Job drawing, mm, ordinate dimensions from the low corner. One solid piece. A direction names the side the tool comes from. Round coordinates to 2 decimals unless told otherwise and drop trailing zeros. Write each loop counter-clockwise with the first axis right and the second up, starting at its lowest first coordinate (ties: lowest second). Pieces come first, ordered by that corner, then holes. Notation, with made-up numbers: M 72.5,16.5 L 86.5,16.5 A34 ccw 86.5,54.5 Z; hole C 13,88 d3. An arc over 180 degrees is marked long. Answer as a JSON object with one key per item and string values. Group by question number.
1. Band-saw the part on D-D, the plane y = 17. Write the cut outline in (x, z), plus the area to 3 significant figures.
2. Band-saw the part on C-C, the plane x = 17.5. Write the cut outline in (y, z), plus the area to 3 significant figures.
3. Band-saw the part on A-A, the plane z = 36. Write the cut outline in (x, y), plus the area to 3 significant figures.
4. Which spindle directions (+Z, -Z, +X, -X, +Y, -Y) get a long thin tool onto all of the face, cutting with end or side? Do the marked faces 3 and 4. Say none if no direction does.
5. Drop flat-ended pins along their axis: pin 1 (4 mm diameter, centred on x = 44, y = 3, fed in from +Z); pin 2 (2.5 mm diameter, centred on x = 62, z = 37, fed in from +Y); pin 3 (2 mm diameter, centred on x = 12, y = 32, fed in from +Z); pin 4 (2 mm diameter, centred on x = 27, y = 6.5, fed in from -Z). Give the stop position or say it passes through.
6. Band-saw the part on B-B, the plane z = 13. Write the cut outline in (x, y).
7. Two-plate mould, pull along X, no slides. Class the marked faces 1 and 2: +X half, -X half, draft (parallel to the pull), parting line (faces both ways), or undercut.
8. Drill centre lines: line 1 (X direction, y = 42, z = 3); line 2 (X direction, y = 28.5, z = 26); line 3 (Y direction, x = 17, z = 1). Where is each one in solid material? Low to high. Write a range as from..to.
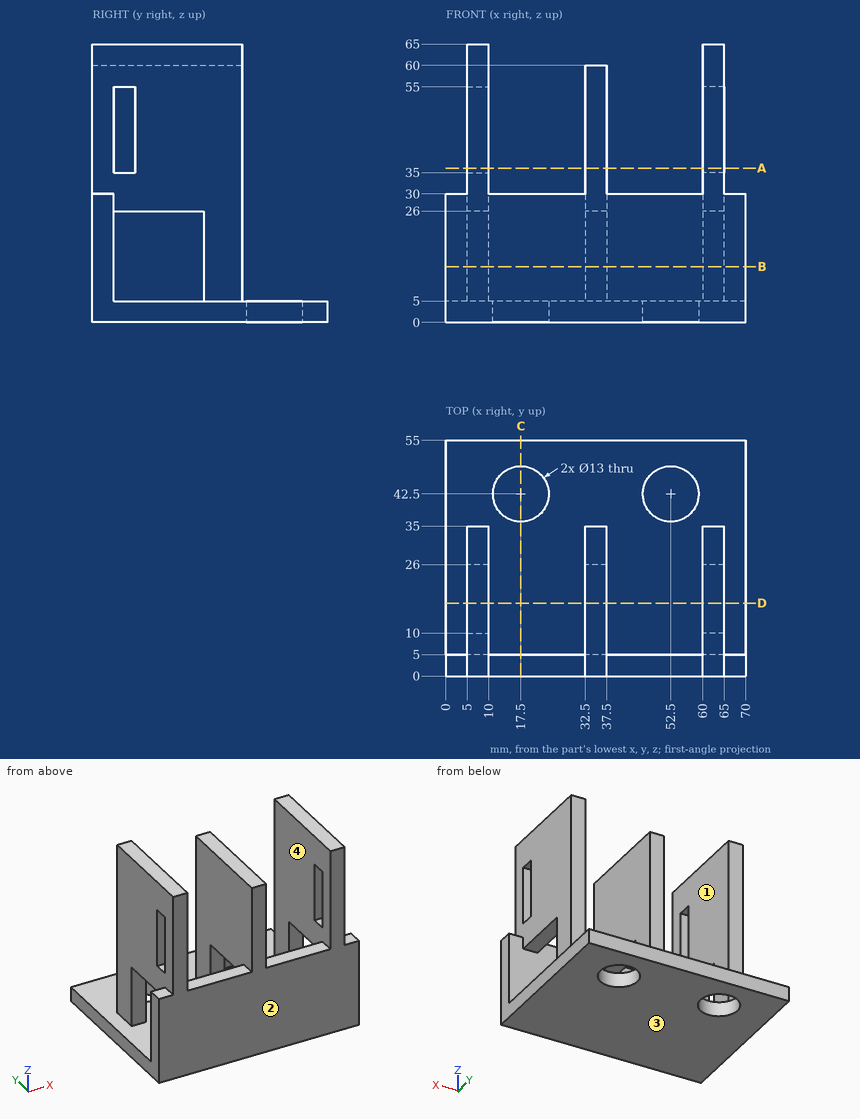
Worked answers:
{
 "1": {"outline": "M 0,0 L 70,0 L 70,5 L 0,5 Z; M 5,26 L 10,26 L 10,65 L 5,65 Z; M 32.5,26 L 37.5,26 L 37.5,60 L 32.5,60 Z; M 60,26 L 65,26 L 65,65 L 60,65 Z", "area": "910 mm^2"},
 "2": {"outline": "M 0,0 L 36,0 L 36,5 L 5,5 L 5,30 L 0,30 Z; M 49,0 L 55,0 L 55,5 L 49,5 Z", "area": "335 mm^2"},
 "3": {"outline": "M 5,0 L 10,0 L 10,5 L 5,5 Z; M 5,10 L 10,10 L 10,35 L 5,35 Z; M 32.5,0 L 37.5,0 L 37.5,35 L 32.5,35 Z; M 60,0 L 65,0 L 65,5 L 60,5 Z; M 60,10 L 65,10 L 65,35 L 60,35 Z", "area": "475 mm^2"},
 "4": {"face 3": "-Z, +X, -X, +Y, -Y", "face 4": "+Z, +Y"},
 "5": {"pin 1": "stops at z = 30", "pin 2": "stops at y = 35", "pin 3": "stops at z = 5", "pin 4": "stops at z = 0"},
 "6": {"outline": "M 0,0 L 70,0 L 70,5 L 0,5 Z; M 5,26 L 10,26 L 10,35 L 5,35 Z; M 32.5,26 L 37.5,26 L 37.5,35 L 32.5,35 Z; M 60,26 L 65,26 L 65,35 L 60,35 Z"},
 "7": {"face 1": "undercut", "face 2": "draft"},
 "8": {"line 1": "x = 0..11.02, 23.98..46.02, 58.98..70", "line 2": "x = 5..10, 32.5..37.5, 60..65", "line 3": "y = 0..36.02, 48.98..55"}
}
